Verification items for this drawing (mm, ordinates from the low corner). A direction names the side the tool comes from. Give positions to 0.01 mm unless a question says otherwise; leave off trailing zeros. Loops run counter-clockwise (first coordinate to the right, second up) from the corner with the lowest first, then second, coordinate; pieces in that order, holes last. Notation, with made-up numbers: (-12, -35) -> (8, -35) arc R26 cw to (8, -7) -> close; hole circle Ø7 at (-36, 59.25). An arc over 180 degrees is marked (long way). Answer in a Markdown table with one row per item. Add a question column.
Q1. Section check B-B on z = 6. Enter the section's corners in (x, y), and give its area (3 significant figures).
Q2. Section check A-A on x = 1. Enter the section's corners in (y, z).
Q3. Section check D-D on z = 23.5. Enter the section's corners in (x, y), and give its area (3 significant figures).
Q4. Set-up check for the marked faces 5 and 6: record each of +Z, -Z, +X, -X, +Y, -Y from which the full face is reachable in a straight line by a thin tool's end or side.
Q5. Gauge pin test, flat ends, axial feed: P1, Ø0.5, axis at x = 2.5, y = 4.5, coming from the -Z side; P2, Ø1.4, axis at x = 2.5, y = 2.5, coming from the +Z side; P3, Ø0.8, axis at x = 4.5, y = 4.5, coming from the -Z side; P4, Ø1.5, axis at x = 2, z = 22.5, coming from the +Y side. Record the tip position at first contact, or that the pin passes through.
Q6. Section check C-C on y = 5.25. Enter the section's corners in (x, z).
Q7. Material ranges on probe 1 along Z at (x, y) = (3.25, 0.5); probe 2 along Z at (x, y) = (4.5, 7); probe 3 along X at (y, z) = (2.75, 22), recorded low to high.
Q8. Release check for a two-part mould opening along Z. For the marked faces 1, 2, 3 and 4 record: pulls with the +Z half, pulls with the -Z half, needs draft (parallel to the pull), parting line crosses it, or undercut.
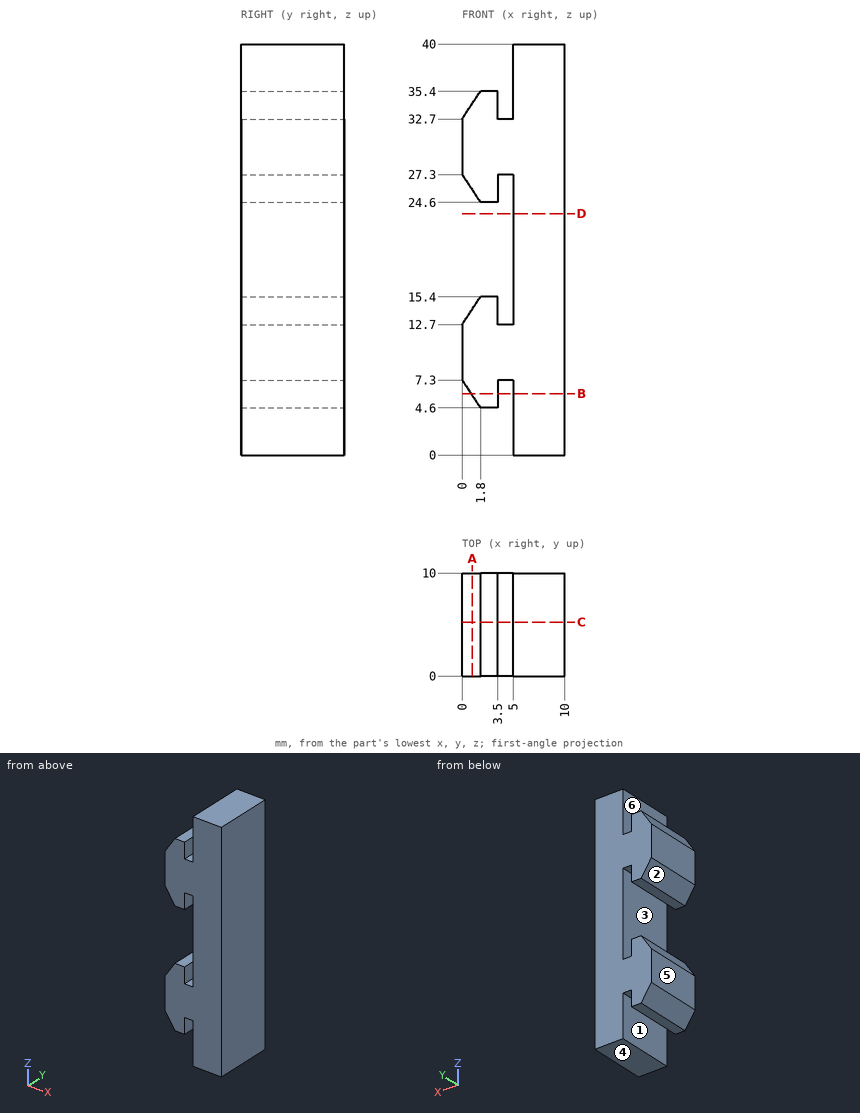
Taken from the geometry:
| question | item | result |
|---|---|---|
| 1 | outline | (0.87, 0) -> (3.5, 0) -> (3.5, 10) -> (0.87, 10) -> close; (5, 0) -> (10, 0) -> (10, 10) -> (5, 10) -> close |
| 1 | area | 76.3 mm² |
| 2 | outline | (0, 5.8) -> (10, 5.8) -> (10, 14.2) -> (0, 14.2) -> close; (0, 25.8) -> (10, 25.8) -> (10, 34.2) -> (0, 34.2) -> close |
| 3 | outline | (5, 0) -> (10, 0) -> (10, 10) -> (5, 10) -> close |
| 3 | area | 50.0 mm² |
| 4 | face 5 | +Z, -Z, -X, +Y, -Y |
| 4 | face 6 | +Z, +Y, -Y |
| 5 | P1 | stops at z = 4.6 |
| 5 | P2 | stops at z = 35.4 |
| 5 | P3 | stops at z = 7.3 |
| 5 | P4 | passes through |
| 6 | outline | (0, 7.3) -> (1.8, 4.6) -> (3.5, 4.6) -> (3.5, 7.3) -> (5, 7.3) -> (5, 0) -> (10, 0) -> (10, 40) -> (5, 40) -> (5, 32.7) -> (3.5, 32.7) -> (3.5, 35.4) -> (1.8, 35.4) -> (0, 32.7) -> (0, 27.3) -> (1.8, 24.6) -> (3.5, 24.6) -> (3.5, 27.3) -> (5, 27.3) -> (5, 12.7) -> (3.5, 12.7) -> (3.5, 15.4) -> (1.8, 15.4) -> (0, 12.7) -> close |
| 7 | probe 1 | z = 4.6 to 15.4, 24.6 to 35.4 |
| 7 | probe 2 | z = 7.3 to 12.7, 27.3 to 32.7 |
| 7 | probe 3 | x = 5 to 10 |
| 8 | face 1 | needs draft |
| 8 | face 2 | undercut |
| 8 | face 3 | undercut |
| 8 | face 4 | pulls with the -Z half |
